Geometry check sheet. Reference: the model listing, model coordinates, mm. A direction names the side the tool comes from. Round coordinates to 2 decimals unless told otherwise and drop trailing zeros. Loops run counter-clockwise (first coordinate to the right, second up) from the corner with the lowest first, then second, coordinate; pieces in that order, holes last. Notation, with made-up numbers: (51, -7.5) -> (83, -7.5) arc R15 cw to (83, -0.5) -> close; hole circle Ø8 at (-33, 29). An arc over 180 degrees is marked (long way). Use one line per item in the form item = value.
from build123d import *

# Parameters (mm, degrees)
F0_R     = 1.75
F0_R_2   = 5.5
F1_DEPTH = 5


# Not quite as in the source:
# - ends of sketch curves that miss each other by under 0.0002 mm in the source are joined


with BuildPart() as f1:
    # F0 (on Top) → F1 (new body)
    with BuildSketch(Plane.XY):
        with BuildLine():
            ThreePointArc((11.3834703749, 6.8633075193), (9.5916723545, 7.355768815), (7.9272258947, 8.1820110654))
            ThreePointArc((7.9272258947, 8.1820110654), (-11.3923753212, 0), (7.9272258947, -8.1820110654))
            ThreePointArc((7.9272258947, -8.1820110654), (9.5459951376, -7.2276126539), (11.3834703749, -6.8339440851))
            Line((11.3834703749, -6.8339440851), (21.8628461179, -6.8339440851))
            ThreePointArc((21.8628461179, -6.8339440851), (24.0780549828, -6.2025675349), (25.9603803998, -4.874923875))
            Line((25.9603803998, -4.874923875), (21.1398675793, -4.874923875))
            ThreePointArc((21.1398675793, -4.874923875), (21.1127528894, -4.8749999983), (21.0856381954, -4.8749253089))
            ThreePointArc((21.0856381954, -4.8749253089), (21.0855085866, -4.8749245897), (21.0853803998, -4.874923875))
            Line((21.0853803998, -4.874923875), (16.2648675793, -4.874923875))
            ThreePointArc((16.2648675793, -4.874923875), (12.9636398268, -3.6120150473), (11.3834703749, -0.4503528446))
            ThreePointArc((11.3834703749, -0.4503528446), (11.3923753212, 0), (11.3834703749, 0.4503528446))
            ThreePointArc((11.3834703749, 0.4503528446), (12.9535739288, 3.6028655537), (16.2376621588, 4.8749999999))
            Line((16.2376621588, 4.8749999999), (21.1319533126, 4.8749616796))
            Line((21.1319533126, 4.8749616796), (25.9603803998, 4.874923875))
            ThreePointArc((25.9603803998, 4.874923875), (23.8013578283, 6.3274272295), (21.2571545841, 6.8734806254))
            Line((21.2571545841, 6.8734806254), (20.9539298759, 6.8731682053))
            Line((20.9539298759, 6.8731682053), (11.3834703749, 6.8633075193))
        make_face()
        with Locations((0, -8)):
            Circle(F0_R, mode=Mode.SUBTRACT)
        with Locations((-8, 0)):
            Circle(F0_R, mode=Mode.SUBTRACT)
        Circle(F0_R_2, mode=Mode.SUBTRACT)
        with Locations((7.9272258947, 0)):
            Circle(F0_R, mode=Mode.SUBTRACT)
        with Locations((0, 8)):
            Circle(F0_R, mode=Mode.SUBTRACT)
    extrude(amount=F1_DEPTH)


solid = f1.part
1. Mould release check, pull along Y, two halves, no side actions. Record for faces 1 (the cylindrical face through (6.18, 0.08, 2.46)), 2 (the flat face through (17, -6.834, 2)), 3 (the flat face through (7, -2, 0)), 4 (the cylindrical face through (-1.19, -5.37, 2.46)): released by +Y, released by -Y, zero draft, split by the parting line, or undercut.
Return value:
face_1 = undercut
face_2 = released by -Y
face_3 = zero draft
face_4 = undercut
2. Section check B-B (x = 0). Record the boundary of the cut face in (y, z).
Return value:
outline = (-11.39, 0) -> (-9.75, 0) -> (-9.75, 5) -> (-11.39, 5) -> close; (-6.25, 0) -> (-5.5, 0) -> (-5.5, 5) -> (-6.25, 5) -> close; (5.5, 0) -> (6.25, 0) -> (6.25, 5) -> (5.5, 5) -> close; (9.75, 0) -> (11.39, 0) -> (11.39, 5) -> (9.75, 5) -> close
3. Gauge pin test, flat ends, axial feed: pin 1 (1.4 mm diameter, centred on x = 18, z = 2, fed in from +Y); pin 2 (2.5 mm diameter, centred on x = 24, z = 2.5, fed in from -Y); pin 3 (5.5 mm diameter, centred on x = -8, y = 0, fed in from +Z); pin 4 (3 mm diameter, centred on x = 0, y = 8, fed in from -Z). Record the tip position at first contact, or that the pin passes through.
Return value:
pin_1 = 6.87
pin_2 = -6.68
pin_3 = 5
pin_4 = through
4. Tool access check on faces 5 (the cylindrical face through (9.616, 7.347, 2.465)), 6 (the flat face through (19, -4.875, 2)). Record the directions out of +Z, -Z, +X, -X, +Y, -Y that give a thin tool (end or side, any length) a straight path to the whole face; none if there is none.
Return value:
face_5 = +Z, -Z, +X, +Y
face_6 = +Z, -Z, +X
5. Section check D-D (x = 12.5). Record the boundary of the cut face in (y, z), then the cut area to 3 significant figures.
Return value:
outline = (-6.83, 0) -> (-3.13, 0) -> (-3.13, 5) -> (-6.83, 5) -> close; (3.13, 0) -> (6.86, 0) -> (6.86, 5) -> (3.13, 5) -> close
area = 37.2 mm2
6. Section check A-A (y = 0). Record the boundary of the cut face in (x, z), then the cut area to 3 significant figures.
Return value:
outline = (-11.39, 0) -> (-9.75, 0) -> (-9.75, 5) -> (-11.39, 5) -> close; (-6.25, 0) -> (-5.5, 0) -> (-5.5, 5) -> (-6.25, 5) -> close; (5.5, 0) -> (6.18, 0) -> (6.18, 5) -> (5.5, 5) -> close; (9.68, 0) -> (11.39, 0) -> (11.39, 5) -> (9.68, 5) -> close
area = 23.9 mm2
7. Section check C-C (z = 4.15). Count the separate pieces of the cut face and the enclosed holes in it, then the cut area to 3 significant figures.
Return value:
separate_pieces = 1
enclosed_holes = 5
area = 348 mm2
8. Material ranges on line 1 along Y through (x, z) = (0, 1.1); line 2 along Y through (x, z) = (-1.5, 3.3); line 3 along Y through (x, z) = (16.5, 1.45) (3 decimals), recorded low to high.
Return value:
line_1 = -11.39 to -9.75, -6.25 to -5.5, 5.5 to 6.25, 9.75 to 11.39
line_2 = -11.29 to -8.9, -7.1 to -5.29, 5.29 to 7.1, 8.9 to 11.29
line_3 = -6.834 to -4.875, 4.875 to 6.869
